CAD build for the part. Positions are in the model's coordinates, mm. A direction names the side the tool comes from. Give positions to 0.01 mm unless a question says otherwise; leave off trailing zeros. Write each loop counter-clockwise with the first axis right and the second up, starting at its lowest first coordinate (ties: lowest second). Pieces come first, ordered by that corner, then holes. Notation, with made-up numbers: (57, 46) - (82, 46) arc R11 cw to (82, 53) - close; hole circle Ø9 at (4.25, 33). An arc over 180 degrees is marked (long way). Put each result on its own line as item: value. Start each with the question number.
1. Cut at D-D on y = 361. List the corners of the cut face in (x, z).
2. Wall check: line 1 (X direction, y = 330.5, z = 162.5); line 2 (Y direction, x = 718.9, z = 184.5); line 3 (Z direction, x = 718.7, y = 335.03). Give the ranges that are in metal, low to high.
3. Cut at A-A on z = 248.02. List the corners of the cut face in (x, y).
4. Tool access for faces 1 (the cylindrical face through (700.01, 339.69, 153.94)), 2 (the cylindrical face through (700.01, 340.82, 202)): list every direction of +Z, -Z, +X, -X, +Y, -Y with a clear straight run to the whole face (end or side of a thin tool).
5. Drop flat-ended pins along their axis: pin 1 (6 mm diameter, centred on x = 715.5, y = 336, fed in from +Z); pin 2 (10 mm diameter, centred on x = 705.5, z = 242.5, fed in from +Y); pin 3 (5 mm diameter, centred on x = 716.5, z = 190.5, fed in from +Y). Give the stop position or say it passes through.
6. Cut at B-B on y = 319.5. List the corners of the cut face in (x, z).
7. Mould opens along Z. For faces 3 (the cylindrical face through (700.01, 356.79, 240.1)), 4 (the flat face through (700.01, 309.1, 162.66)), 5 (the flat face through (719.009, 321.007, 225.654)) say: +Z half, -Z half, draft (parallel to the pull), parting line (faces both ways), or undercut.
8. Cut at C-C on x = 705. List the corners of the cut face in (y, z), and give its area (3 significant figures).
from build123d import *

# Parameters (mm, degrees)
SKETCH1_R               = 4
SKETCH1_R_2             = 11
BOSS_EXTRUDE2_DEPTH     = 11
SKETCH1_8_R             = 4
CUT_EXTRUDE1_DEPTH      = 8
CUT_EXTRUDE2_DEPTH      = 1
CUT_EXTRUDE2_DEPTH_BACK = 23
SKETCH6_R               = 4
BOSS_EXTRUDE8_DEPTH     = 11
SKETCH6_6_R             = 4
CUT_EXTRUDE3_DEPTH      = 8


with BuildPart() as part:
    # Sketch1 → Boss-Extrude2 (new body, symmetric)
    with BuildSketch(Plane.ZY.offset(-709.53)):
        with BuildLine():
            Line((193.569972926, 283.579288774), (258.649201612, 359.498464834))
            ThreePointArc((258.649201612, 359.498464834), (258.8956606, 377.425895105), (241.305287216, 380.894650269))
            Line((241.305287216, 380.894650269), (178.264909558, 346.43717525))
            ThreePointArc((178.264909558, 346.43717525), (173.380579242, 341.764870601), (171.502250327, 335.271874849))
            Line((171.502250327, 335.271874849), (170.702250327, 292.281874849))
            ThreePointArc((170.702250327, 292.281874849), (179.076203082, 279.89008222), (193.569972926, 283.579288774))
        make_face()
        with Locations((248.02, 368.61)):
            Circle(SKETCH1_R, mode=Mode.SUBTRACT)
        with Locations((184.5, 335.03)):
            Circle(SKETCH1_R, mode=Mode.SUBTRACT)
        with Locations((183.7, 292.04)):
            Circle(SKETCH1_R_2, mode=Mode.SUBTRACT)
    extrude(amount=BOSS_EXTRUDE2_DEPTH, both=True)

    # Sketch1_8 → Cut-Extrude1 (cut, symmetric)
    with BuildSketch(Plane.ZY.offset(-709.53)):
        with BuildLine():
            Line((193.569972926, 283.579288774), (258.649201612, 359.498464834))
            ThreePointArc((258.649201612, 359.498464834), (258.8956606, 377.425895105), (241.305287216, 380.894650269))
            Line((241.305287216, 380.894650269), (178.264909558, 346.43717525))
            ThreePointArc((178.264909558, 346.43717525), (173.380579242, 341.764870601), (171.502250327, 335.271874849))
            Line((171.502250327, 335.271874849), (170.702250327, 292.281874849))
            ThreePointArc((170.702250327, 292.281874849), (188.323796918, 304.18991778), (193.569972926, 283.579288774))
        make_face()
        with Locations((248.02, 368.61)):
            Circle(SKETCH1_8_R, mode=Mode.SUBTRACT)
        with Locations((184.5, 335.03)):
            Circle(SKETCH1_8_R, mode=Mode.SUBTRACT)
    extrude(amount=CUT_EXTRUDE1_DEPTH, both=True, mode=Mode.SUBTRACT)

    # Sketch5 → Cut-Extrude2 (cut, two sides)
    with BuildSketch(Plane.ZY.offset(-698.53)) as cut_extrude2_sk:
        with BuildLine():
            Line((231.673739179, 358.535602781), (205.718398062, 344.348576127))
            ThreePointArc((205.718398062, 344.348576127), (201.961220896, 340.754495628), (200.5163525, 335.75988351))
            Line((200.5163525, 335.75988351), (200.141351056, 315.608243405))
            ThreePointArc((200.141351056, 315.608243405), (203.362102115, 310.842169317), (208.936628978, 312.261094915))
            Line((208.936628978, 312.261094915), (239.902269766, 348.384539863))
            ThreePointArc((239.902269766, 348.384539863), (240.019198117, 356.889909813), (231.673739179, 358.535602781))
        make_face()
    extrude(amount=CUT_EXTRUDE2_DEPTH, mode=Mode.SUBTRACT)
    extrude(cut_extrude2_sk.sketch, amount=-CUT_EXTRUDE2_DEPTH_BACK, mode=Mode.SUBTRACT)

    # Sketch6 → Boss-Extrude8 (add, symmetric)
    with BuildSketch(Plane.ZY.offset(-709.53)):
        with BuildLine():
            ThreePointArc((160.253054899, 346.051184701), (153.890022283, 339.565239259), (153.896376335, 330.479226273))
            Line((153.896376335, 330.479226273), (171.671074363, 287.109995129))
            ThreePointArc((171.671074363, 287.109995129), (170.922257468, 289.64640526), (170.702250327, 292.281874849))
            Line((170.702250327, 292.281874849), (171.502250327, 335.271874849))
            ThreePointArc((171.502250327, 335.271874849), (173.380579242, 341.764870601), (178.264909558, 346.43717525))
            Line((178.264909558, 346.43717525), (241.305287216, 380.894650269))
            ThreePointArc((241.305287216, 380.894650269), (241.886887594, 381.195107557), (242.481897383, 381.468048818))
            Line((242.481897383, 381.468048818), (160.253054899, 346.051184701))
        make_face()
        with Locations((165, 335.03)):
            Circle(SKETCH6_R, mode=Mode.SUBTRACT)
    extrude(amount=BOSS_EXTRUDE8_DEPTH, both=True)

    # Sketch6_6 → Cut-Extrude3 (cut, symmetric)
    with BuildSketch(Plane.ZY.offset(-709.53)):
        with BuildLine():
            ThreePointArc((160.253054899, 346.051184701), (153.890022283, 339.565239259), (153.896376335, 330.479226273))
            Line((153.896376335, 330.479226273), (171.671074363, 287.109995129))
            ThreePointArc((171.671074363, 287.109995129), (170.922257468, 289.64640526), (170.702250327, 292.281874849))
            Line((170.702250327, 292.281874849), (171.502250327, 335.271874849))
            ThreePointArc((171.502250327, 335.271874849), (173.380579242, 341.764870601), (178.264909558, 346.43717525))
            Line((178.264909558, 346.43717525), (241.305287216, 380.894650269))
            ThreePointArc((241.305287216, 380.894650269), (241.886887594, 381.195107557), (242.481897383, 381.468048818))
            Line((242.481897383, 381.468048818), (160.253054899, 346.051184701))
        make_face()
        with Locations((165, 335.03)):
            Circle(SKETCH6_6_R, mode=Mode.SUBTRACT)
    extrude(amount=CUT_EXTRUDE3_DEPTH, both=True, mode=Mode.SUBTRACT)


solid = part.part
Report:
1. outline: (698.53, 194.96) - (701.53, 194.96) - (701.53, 259.77) - (698.53, 259.77) - close; (717.53, 194.96) - (720.53, 194.96) - (720.53, 259.77) - (717.53, 259.77) - close
2. line 1: x = 698.53 to 701.53, 717.53 to 720.53
2. line 2: y = 279.06 to 281.07, 303.01 to 331.03, 339.03 to 356.49
2. line 3: z = 153 to 161, 169 to 180.5, 188.5 to 200.5, 228.45 to 237.67
3. outline: (698.53, 347.1) - (701.53, 347.1) - (701.53, 364.61) - (698.53, 364.61) - close; (698.53, 372.61) - (701.53, 372.61) - (701.53, 382.61) - (698.53, 382.61) - close; (717.53, 347.1) - (720.53, 347.1) - (720.53, 364.61) - (717.53, 364.61) - close; (717.53, 372.61) - (720.53, 372.61) - (720.53, 382.61) - (717.53, 382.61) - close
4. face 1: -Z, +X, -X
4. face 2: +X, -X
5. pin 1: stops at z = 240.4
5. pin 2: stops at y = 382.39
5. pin 3: stops at y = 360.06
6. outline: (698.53, 158.4) - (701.53, 158.4) - (701.53, 200.21) - (698.53, 200.21) - close; (698.53, 215.14) - (701.53, 215.14) - (701.53, 224.36) - (698.53, 224.36) - close; (717.53, 158.4) - (720.53, 158.4) - (720.53, 200.21) - (717.53, 200.21) - close; (717.53, 215.14) - (720.53, 215.14) - (720.53, 224.36) - (717.53, 224.36) - close
7. face 3: undercut
7. face 4: -Z half
7. face 5: +Z half
8. outline: circle Ø26 at (292.04, 183.7); hole circle Ø22 at (292.04, 183.7)
8. area: 151 mm²
